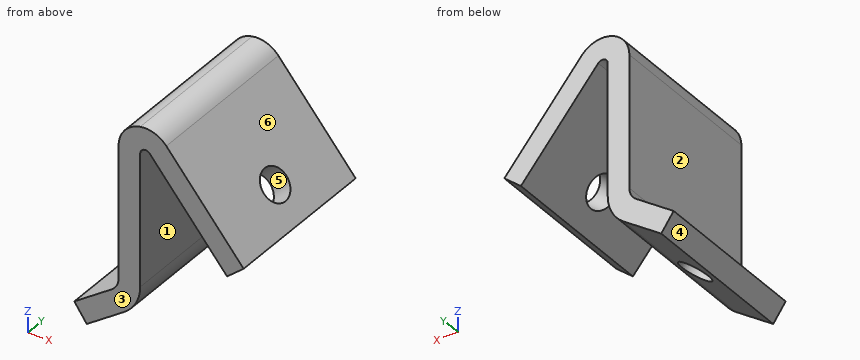
```python
from build123d import *

# Parameters (mm, degrees)
SKETCH_2_W                       = 35
SKETCH_2_H                       = 30
EXTRUDE_1_DEPTH                  = 1
SHEET_START                      = -35
SHEET_METAL_1_OUTLINE_W          = 3
SHEET_METAL_1_OUTLINE_H          = 30
SHEET_METAL_1_DEPTH              = 35
SM_EDGE_FLANGE_1_DEPTH           = 30
SM_EDGE_FLANGE_1_2_DEPTH         = 30
SM_EDGE_FLANGE_2_STRIP_CUT_DEPTH = 30
SM_EDGE_FLANGE_2_DEPTH           = 30
SM_START                         = 4
SM_EDGE_FLANGE_2_PROFILE_W       = 30
SM_EDGE_FLANGE_2_PROFILE_H       = 8.438298848
SM_EDGE_FLANGE_2_PROFILE_R       = 3
SM_EDGE_FLANGE_2_FLAT_DEPTH      = 4
CUT_EXTRUDE_1_REACH              = 58.3
SKETCH_20_R                      = 3
SCALE_1_SCALE                    = 0.3


# Read off the part's stored shape, not the designer's step: 转换实体1, 边线-法兰1
# Sheet-metal steps are written as plain solids
with BuildPart() as part:
    # Sketch 2 → 凸台-拉伸1 (new body)
    with BuildSketch(Plane(origin=(0, 0, 0), x_dir=(0, 0, -1), z_dir=(1, 0, 0))):
        with Locations((17.5, 15)):
            Rectangle(SKETCH_2_W, SKETCH_2_H)
    extrude(amount=EXTRUDE_1_DEPTH)

    # Sheet Metal 1 outline → Sheet Metal 1 (add)
    with BuildSketch(Plane.XY.offset(SHEET_START)):
        with Locations((-1.5, 15)):
            Rectangle(SHEET_METAL_1_OUTLINE_W, SHEET_METAL_1_OUTLINE_H)
    extrude(amount=SHEET_METAL_1_DEPTH)

    # 边线-法兰1 outline → 边线-法兰1 (cut)
    with BuildSketch(Plane(origin=(0, 0, 0), x_dir=(1, 0, 0), z_dir=(0, 1, 0))):
        with BuildLine():
            Line((1, 0), (1, 4.071393241))
            ThreePointArc((1, 4.071393241), (-1.872983346, 5.808095067), (-3, 8.970372727))
            Line((-3, 8.970372727), (-3, 0))
            Line((-3, 0), (1, 0))
        make_face()
    extrude(amount=SM_EDGE_FLANGE_1_DEPTH, mode=Mode.SUBTRACT)

    # Sm Edge Flange 1 2 outline → Sm Edge Flange 1 2 (add)
    with BuildSketch(Plane(origin=(0, 0, 0), x_dir=(1, 0, 0), z_dir=(0, 1, 0))):
        with BuildLine():
            ThreePointArc((1, 4.071393241), (3.646930663, 4.249396197), (5.830222216, 5.756434678))
            Line((5.830222216, 5.756434678), (20.133868015, 22.802855947))
            Line((20.133868015, 22.802855947), (17.069690242, 25.374006385))
            Line((17.069690242, 25.374006385), (2.766044443, 8.327585117))
            ThreePointArc((2.766044443, 8.327585117), (1.657979857, 8.030680106), (1, 8.970372727))
            Line((1, 8.970372727), (1, 4.071393241))
        make_face()
    extrude(amount=SM_EDGE_FLANGE_1_2_DEPTH)

    # 边线-法兰2 strip (across the edge) → 边线-法兰2 strip cut (cut)
    with BuildSketch(Plane(origin=(-3, 30, -35), x_dir=(-0.5735764363510502, 0, 0.8191520442889889), z_dir=(0, -1, 0))):
        Polygon((-19.036380029, 8.446318441), (-1.015035054, -4.172363158), (1.279270691, -0.895754981), (-16.742074283, 11.722926619), align=None)
    extrude(amount=SM_EDGE_FLANGE_2_STRIP_CUT_DEPTH, mode=Mode.SUBTRACT)

    # 边线-法兰2 bend section (across the edge) → 边线-法兰2 (add)
    with BuildSketch(Plane(origin=(-3, 30, -35), x_dir=(-0.5735764363510502, 0, 0.8191520442889889), z_dir=(0, -1, 0))):
        with BuildLine():
            Line((-4, 1.561701152), (0, 1.561701152))
            ThreePointArc((0, 1.561701152), (0.3389675, 0.176455312), (1.279270691, -0.895754981))
            Line((1.279270691, -0.895754981), (-1.015035054, -4.172363158))
            ThreePointArc((-1.015035054, -4.172363158), (-3.209075832, -1.670539141), (-4, 1.561701152))
        make_face()
    extrude(amount=SM_EDGE_FLANGE_2_DEPTH)

    # 边线-法兰2 profile (on flange) → 边线-法兰2 flat (add)
    with BuildSketch(Plane(origin=(-3, 0, -35), x_dir=(0, -1, 0), z_dir=(0.5735764363510502, 0, -0.8191520442889889)).offset(SM_START)):
        with Locations((-15, 5.780850576)):
            Rectangle(SM_EDGE_FLANGE_2_PROFILE_W, SM_EDGE_FLANGE_2_PROFILE_H)
        with Locations((-15, 5)):
            Circle(SM_EDGE_FLANGE_2_PROFILE_R, mode=Mode.SUBTRACT)
    extrude(amount=-SM_EDGE_FLANGE_2_FLAT_DEPTH)

    # 草图20 → 切除-拉伸1 (cut, up to next)
    with BuildSketch(Plane(origin=(-2.477353684, 0, -2.078746562), x_dir=(-0.6427876096865404, 0, 0.7660444431189772), z_dir=(-0.7660444431189772, 0, -0.6427876096865404)), mode=Mode.PRIVATE) as cut_extrude_1_sk1:
        with Locations((-23.351124779, 15)):
            Circle(SKETCH_20_R)
    cut_extrude_1_tool1 = extrude(cut_extrude_1_sk1.sketch, amount=-CUT_EXTRUDE_1_REACH, mode=Mode.PRIVATE) & part.part
    add(cut_extrude_1_tool1.solids().sort_by_distance((12.53246, 15, -19.966746))[0], mode=Mode.SUBTRACT)


with BuildPart() as part_1:
    # 缩放比例1: scaled about (2.566692586, 15, -20.896699523)
    add(part.part.scale(SCALE_1_SCALE).moved(Location((1.79668481, 10.5, -14.627689666))))


solid = part_1.part
```
Verification items for the finished model (mm, model axes). Face numbers are marked on the shaded views. A direction names the side the tool comes from. Coordinates: 2 decimals unless noted, no trailing zeros. Order: outer loops, then holes, each group sorted by start corner. A loop starts at its lowest first (then second) coordinate and runs counter-clockwise, first axis right, second up. Notation, with made-up numbers: (10.25, -1.5) - (49.25, -1.5) arc R10 cw to (49.25, 2.5) - close; hole circle Ø2 at (-16, 55.5). An arc over 180 degrees is marked (long way). Return JSON: item names as keys, results as strings.
(1) Section check A-A, the plane y = 15.75. Record the cut outline in (x, z).
Filled sheet:
{"outline": "(-1.56, -26.85) - (-0.87, -27.83) - (-0.05, -27.26) - (-0.74, -26.27) - close; (0.08, -25.7) - (0.76, -26.69) - (1.2, -26.38) arc R2.1 ccw to (2.1, -24.66) - (2.1, -17.32) arc R0.3 cw to (2.63, -17.13) - (5.24, -20.24) - (6.16, -19.47) - (3.55, -16.35) arc R1.5 ccw to (0.9, -17.32) - (0.9, -24.66) arc R0.9 cw to (0.51, -25.4) - close; (5.88, -21) - (6.92, -22.24) - (7.84, -21.47) - (6.8, -20.23) - close"}
(2) Section check B-B, the plane y = 18. Record the cut outline in (x, z).
Filled sheet:
{"outline": "(-1.56, -26.85) - (-0.87, -27.83) - (1.2, -26.38) arc R2.1 ccw to (2.1, -24.66) - (2.1, -17.32) arc R0.3 cw to (2.63, -17.13) - (6.92, -22.24) - (7.84, -21.47) - (3.55, -16.35) arc R1.5 ccw to (0.9, -17.32) - (0.9, -24.66) arc R0.9 cw to (0.51, -25.4) - close"}
(3) Mould release check, pull along Z, two halves, no side actions. Record for the marked faces 4, 5 and 6: pulls with the +Z half, pulls with the -Z half, needs draft (parallel to the pull), parting line crosses it, or undercut.
Filled sheet:
{"face 4": "pulls with the -Z half", "face 5": "undercut", "face 6": "pulls with the +Z half"}
(4) Section check C-C, the plane z = -18. Record the cut outline in (x, y).
Filled sheet:
{"outline": "(0.9, 10.5) - (2.1, 10.5) - (2.1, 19.5) - (0.9, 19.5) - close; (3.36, 10.5) - (4.93, 10.5) - (4.93, 19.5) - (3.36, 19.5) - close"}
(5) Thickness scan on line 1 along X through (y, z) = (16, -21.25); line 2 along X through (y, z) = (12.75, -20); line 3 along X through (y, z) = (16, -23). Record the ranges inside material, lowest first.
Filled sheet:
{"line 1": "x = 0.9 to 2.1, 6.09 to 7.65", "line 2": "x = 0.9 to 2.1, 5.04 to 6.6", "line 3": "x = 0.9 to 2.1"}
(6) Section check D-D, the plane x = 1.5. Record the cut outline in (y, z).
Filled sheet:
{"outline": "(10.5, -26.13) - (19.5, -26.13) - (19.5, -16.12) - (10.5, -16.12) - close"}
(7) Access from +Z, -Z, +X, -X, +Y, -Y to the whole of each face (thin tool, end or side, straight path). Record for the marked faces 1, 2 and 3.
Filled sheet:
{"face 1": "-Z, +Y, -Y", "face 2": "+Z, -X, +Y, -Y", "face 3": "+Z, -Z, +X, -X, -Y"}
(8) Go/stop test with flat-tipped pins: pin 1 (4 mm diameter, centred on x = 1.5, y = 13, fed in from -Z); pin 2 (2 mm diameter, centred on y = 14.5, z = -21.5, fed in from -X); pin 3 (5 mm diameter, centred on x = 5.5, y = 15.5, fed in from +Z); pin 4 (3.5 mm diameter, centred on y = 14.5, z = -21, fed in from +X). Record where each tip stops, or that it passes through.
Filled sheet:
{"pin 1": "stops at z = -27.57", "pin 2": "stops at x = 0.9", "pin 3": "stops at z = -15.95", "pin 4": "stops at x = 7.84"}
